Part model, mm, in its own coordinate system. Face numbers are marked on the shaded views. A direction names the side the tool comes from. Give positions to 0.01 mm unless a question says otherwise; leave off trailing zeros. Write each loop counter-clockwise with the first axis right and the second up, starting at its lowest first coordinate (ties: lowest second). Pieces come first, ordered by that corner, then holes.
```python
from build123d import *

# Parameters (mm, degrees)
BOSS_EXTRUDE1_DEPTH = 130
SKETCH2_W           = 120
SKETCH2_H           = 132.917960675
BOSS_EXTRUDE2_DEPTH = 80
SKETCH3_R           = 5
CUT_EXTRUDE1_DEPTH  = 68.082039325
CUT_EXTRUDE3_DEPTH  = 40
CHAMFER1_SIZE       = 5
FILLET1_R           = 6
CUT_EXTRUDE4_DEPTH  = 41
SKETCH6_W           = 84.22291236
SKETCH6_H           = 130.917960675
CUT_EXTRUDE5_DEPTH  = 25


with BuildPart() as part:
    # Sketch1 → Boss-Extrude1 (new body)
    with BuildSketch(Plane.XY):
        Polygon((0, 0), (-60, 67.082039325), (60, 67.082039325), align=None)
        Polygon((0, 12), (-42.11145618, 59.082039325), (42.11145618, 59.082039325), align=None, mode=Mode.SUBTRACT)
    extrude(amount=BOSS_EXTRUDE1_DEPTH)

    # Sketch2 → Boss-Extrude2 (add)
    with BuildSketch(Plane(origin=(0, 0, 0), x_dir=(-1, 0, 0), z_dir=(0, 0, -1))):
        with Locations((0, 133.541019662)):
            Rectangle(SKETCH2_W, SKETCH2_H)
    extrude(amount=-BOSS_EXTRUDE2_DEPTH)

    # Sketch3 → Cut-Extrude1 (cut, through all)
    with BuildSketch(Plane(origin=(0, 67.082039325, 0), x_dir=(1, 0, 0), z_dir=(0, 1, 0))):
        with Locations((0, -110)):
            Circle(SKETCH3_R)
    extrude(amount=-CUT_EXTRUDE1_DEPTH, mode=Mode.SUBTRACT)

    # Sketch4 → Cut-Extrude3 (cut)
    with BuildSketch(Plane.XY.offset(80)):
        with BuildLine():
            Line((-40, 200), (-40, 120))
            ThreePointArc((-40, 120), (0, 80), (40, 120))
            Line((40, 120), (40, 200))
            Line((40, 200), (-40, 200))
        make_face()
    extrude(amount=-CUT_EXTRUDE3_DEPTH, mode=Mode.SUBTRACT)

    # Chamfer1
    chamfer1_edges = [part.edges().sort_by_distance(p)[0] for p in [
        (-40, 160, 80),
        (0, 80, 80),
        (40, 160, 80),
    ]]
    chamfer(chamfer1_edges, length=CHAMFER1_SIZE)

    # Fillet1
    fillet1_edges = [part.edges().sort_by_distance(p)[0] for p in [
        (0, 67.082039325, 80),
    ]]
    fillet(fillet1_edges, radius=FILLET1_R)

    # Sketch5 → Cut-Extrude4 (cut, through all)
    with BuildSketch(Plane.XY.offset(40)):
        with BuildLine():
            Line((10, 170), (10, 120))
            ThreePointArc((10, 120), (0, 110), (-10, 120))
            Line((-10, 120), (-10, 170))
            ThreePointArc((-10, 170), (0, 180), (10, 170))
        make_face()
    extrude(amount=-CUT_EXTRUDE4_DEPTH, mode=Mode.SUBTRACT)

    # Sketch6 → Cut-Extrude5 (cut)
    with BuildSketch(Plane(origin=(0, 0, 0), x_dir=(-1, 0, 0), z_dir=(0, 0, -1))):
        with Locations((0, 124.541019663)):
            Rectangle(SKETCH6_W, SKETCH6_H)
    extrude(amount=-CUT_EXTRUDE5_DEPTH, mode=Mode.SUBTRACT)


solid = part.part
```
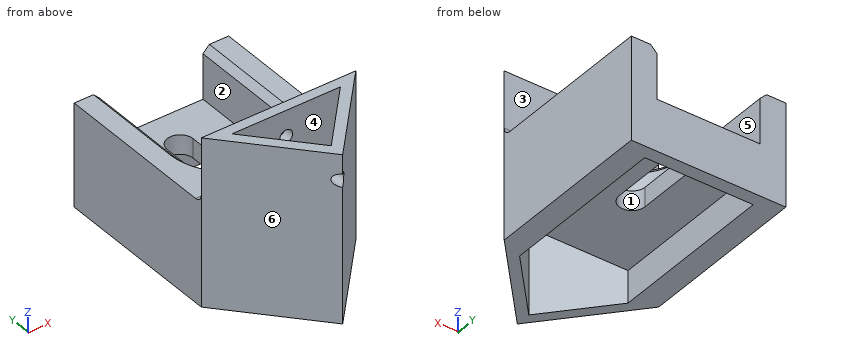
1) Wall check: L1, parallel to Z at x = 0, y = 65; L2, parallel to X at y = 152, z = 23; L3, parallel to Z at x = 0, y = 7.75. Give the ranges that are in metal, low to high.
Answers follow:
L1: z = 25 to 105, 115 to 130
L2: x = -60 to -42.11, 42.11 to 60
L3: z = 0 to 105, 115 to 130
2) Saw through at C-C, the plane z = 13. Write the cut outline in (x, y), then the cut area to 3 significant figures.
Answers follow:
outline: (-60, 67.08) - (0, 0) - (60, 67.08) - (60, 200) - (-60, 200) - close; hole (-42.11, 59.08) - (0, 12) - (42.11, 59.08) - (42.11, 190) - (-42.11, 190) - close
area: 6,970 mm2
3) Pin check, flat tips, straight feed: pin 1 Ø3 at (x, z) = (-33, 42.5) entering from -Y; pin 2 Ø12 at (x, z) = (21, 76) entering from -Y; pin 3 Ø8 at (x, z) = (-7, 114.5) entering from -Y; pin 4 Ø16 at (x, z) = (0, 110) entering from -Y. Stop position of each tip, or through.
Answers follow:
pin 1: stops at y = 35.22
pin 2: stops at y = 16.77
pin 3: stops at y = 3.35
pin 4: stops at y = 0
4) Two-plate mould, pull along Y, no slides. Class the marked faces 4, 5 and 6: +Y half, -Y half, draft (parallel to the pull), parting line (faces both ways), or undercut.
Answers follow:
face 4: undercut
face 5: draft
face 6: -Y half
5) Saw through at B-B, the plane z = 49. Write the cut outline in (x, y).
Answers follow:
outline: (-60, 67.08) - (0, 0) - (60, 67.08) - (60, 200) - (40, 200) - (40, 120) arc R40 cw to (-40, 120) - (-40, 200) - (-60, 200) - close; hole (-42.11, 59.08) - (0, 12) - (42.11, 59.08) - close
6) Saw through at A-A, the plane y = 135. Write the cut outline in (x, z), then the cut area to 3 significant figures.
Answers follow:
outline: (-60, 0) - (-42.11, 0) - (-42.11, 25) - (-10, 25) - (-10, 40) - (-40, 40) - (-40, 75) - (-45, 80) - (-60, 80) - close; (10, 25) - (42.11, 25) - (42.11, 0) - (60, 0) - (60, 80) - (45, 80) - (40, 75) - (40, 40) - (10, 40) - close
area: 3,970 mm2
7) Saw through at D-D, the plane z = 90. Write the cut outline in (x, y), then the cut area to 3 significant figures.
Answers follow:
outline: (-60, 67.08) - (0, 0) - (60, 67.08) - close; hole (-42.11, 59.08) - (0, 12) - (42.11, 59.08) - close
area: 2,040 mm2
8) 3-axis set-ups, long thin cutter, end or side, ignore diameter. For the marked faces 1, 2 and 3: which of +Z, -Z, +X, -X, +Y, -Y reach the whole face in a straight line?
Answers follow:
face 1: +Z, -Z
face 2: +Z, +Y
face 3: +Z, +X, -X, +Y
